Part model, mm, in its own coordinate system. Face numbers are marked on the shaded views. A direction names the side the tool comes from. Round coordinates to 2 decimals unless told otherwise and drop trailing zeros. Write each loop counter-clockwise with the first axis right and the second up, starting at its lowest first coordinate (ties: lowest second). Pieces come first, ordered by that corner, then holes.
from build123d import *

# Parameters (mm, degrees)
SCHIZZO1_R                        = 10
ESTRUSIONE_ESTRUSIONE1_DEPTH      = 20
ESTRUSIONE_ESTRUSIONE2_DEPTH      = 8
ESTRUSIONE_ESTRUSIONE2_DEPTH_BACK = 8
SCHIZZO3_R                        = 8
TAGLIO_ESTRUSIONE1_DEPTH          = 20
SCHIZZO4_R                        = 3.75
TAGLIO_ESTRUSIONE2_DEPTH          = 8
RACCORDO1_R                       = 2
TAGLIO_ESTRUSIONE4_REACH          = 20
RACCORDO4_R                       = 3


with BuildPart() as part:
    # Schizzo1 → Estrusione-Estrusione1 (new body)
    with BuildSketch(Plane.XY):
        Circle(SCHIZZO1_R)
    extrude(amount=ESTRUSIONE_ESTRUSIONE1_DEPTH)

    # Schizzo2 → Estrusione-Estrusione2 (add, two sides)
    with BuildSketch(Plane(origin=(0, 0, 0), x_dir=(0, 0, -1), z_dir=(1, 0, 0))) as estrusione_estrusione2_sk:
        Polygon((0, 0), (-20, 0), (-20, -14), (-46, -14), (-46, 0), (-61, 0), (-61, -51.86222015), (-21.859762995, -51.86222015), (0, -14), align=None)
    extrude(amount=ESTRUSIONE_ESTRUSIONE2_DEPTH)
    extrude(estrusione_estrusione2_sk.sketch, amount=-ESTRUSIONE_ESTRUSIONE2_DEPTH_BACK)

    # Schizzo3 → Taglio-Estrusione1 (cut)
    with BuildSketch(Plane(origin=(0, 0, 0), x_dir=(-1, 0, 0), z_dir=(0, 0, -1))):
        Circle(SCHIZZO3_R)
    extrude(amount=-TAGLIO_ESTRUSIONE1_DEPTH, mode=Mode.SUBTRACT)

    # Schizzo4 → Taglio-Estrusione2 (cut)
    with BuildSketch(Plane.XZ.offset(51.86222015)):
        with Locations((0, 38)):
            Circle(SCHIZZO4_R)
    extrude(amount=-TAGLIO_ESTRUSIONE2_DEPTH, mode=Mode.SUBTRACT)

    # Raccordo1
    raccordo1_edges = [part.edges().sort_by_distance(p)[0] for p in [
        (8, -10, 20),
        (8, -14, 33),
        (8, -7, 46),
        (8, 0, 53.5),
        (8, -25.931110075, 61),
        (8, -51.86222015, 41.429881498),
        (8, -32.931110075, 10.929881498),
        (0, -14, 0),
        (-8, -32.931110075, 10.929881498),
        (0, -51.86222015, 21.859762995),
        (-8, -51.86222015, 41.429881498),
        (0, -51.86222015, 61),
        (-8, -25.931110075, 61),
        (0, 0, 61),
        (-8, 0, 53.5),
        (0, 0, 46),
        (-8, -7, 46),
        (0, -14, 46),
        (-8, -14, 33),
        (-8, -10, 20),
        (0, -14, 20),
        (-3.75, -51.86222015, 38),
    ]]
    fillet(raccordo1_edges, radius=RACCORDO1_R)

    # Schizzo6 → Taglio-Estrusione4 (cut, up to next)
    with BuildSketch(Plane(origin=(8, 0, 0), x_dir=(0, 0, -1), z_dir=(1, 0, 0)), mode=Mode.PRIVATE) as taglio_estrusione4_sk1:
        Polygon((-54, -21), (-12.124355653, -21), (-21.282412726, -36.86222015), (-54, -36.86222015), align=None)
    taglio_estrusione4_tool1 = extrude(taglio_estrusione4_sk1.sketch, amount=-TAGLIO_ESTRUSIONE4_REACH, mode=Mode.PRIVATE) & part.part
    add(taglio_estrusione4_tool1.solids().sort_by_distance((8, -28.606534, 35.257995))[0], mode=Mode.SUBTRACT)

    # Raccordo4
    raccordo4_edges = [part.edges().sort_by_distance(p)[0] for p in [
        (0, -36.86222015, 54),
        (0, -21, 54),
        (0, -21, 12.124355653),
        (0, -36.86222015, 21.282412726),
        (8, -28.931110075, 54),
        (8, -36.86222015, 37.641206363),
        (8, -28.931110075, 16.70338419),
        (8, -21, 33.062177826),
        (-8, -36.86222015, 37.641206363),
        (-8, -28.931110075, 54),
        (-8, -21, 33.062177826),
        (-8, -28.931110075, 16.70338419),
    ]]
    fillet(raccordo4_edges, radius=RACCORDO4_R)


solid = part.part
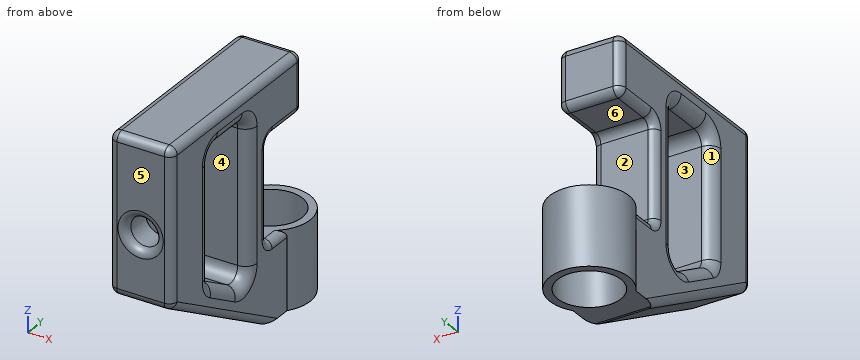
Q1. Drop flat-ended pins along their axis: P1, Ø7, axis at x = 0, z = 38, coming from the +Y side; P2, Ø5, axis at y = -30, z = 12, coming from the +X side; P3, Ø12, axis at x = -1, y = -21, coming from the -Z side; P4, Ø5, axis at x = -7, z = 30, coming from the -Y side. Give the stop position or say it passes through.
Q2. Saw through at A-A, the plane x = 0. Give the number of separate pieces and of enclosed holes in the cut face, and give its area (3 significant figures).
Q3. Two-plate mould, pull along Y, no slides. Class the marked faces 4, 5 and 6: released by +Y, released by -Y, zero draft, split by the parting line, or undercut.
Q4. Saw through at B-B, the plane y = 1. Write the cut outline in (x, z), and give its area (3 significant figures).
Q5. Tool access for the marked faces 1, 2 and 3: list every direction of +Z, -Z, +X, -X, +Y, -Y with a clear straight run to the whole face (end or side of a thin tool).
Q6. Wall check: line 1 (Y direction, x = -2.5, z = 25); line 2 (Y direction, x = 6.5, z = 15); line 3 (Y direction, x = 3, z = 49.5). Give the ranges that are in metal, low to high.
Computed:
1. P1: stops at y = -14
1. P2: stops at x = 8
1. P3: stops at z = 0.58
1. P4: stops at y = -51.86
2. separate pieces: 2
2. enclosed holes: 1
2. area: 1,620 mm2
3. face 4: undercut
3. face 5: released by -Y
3. face 6: zero draft
4. outline: (-9.95, 0) - (-7.94, 0) - (-7.94, 20) - (-9.95, 20) - close; (7.94, 0) - (9.95, 0) - (9.95, 20) - (7.94, 20) - close
4. area: 80.5 mm2
5. face 1: -X
5. face 2: +X, -X, +Y
5. face 3: +X, -X
6. line 1: y = -51.86 to -36.86, -21 to -14
6. line 2: y = -39.85 to -26.78, -21.51 to -4.66, 4.66 to 7.6
6. line 3: y = -51.86 to -36.86, -21 to 0
